Here's how the part is built. I have some questions about the finished solid (model axes, mm). Round coordinates to 2 decimals unless told otherwise and drop trailing zeros. Order: outer loops, then holes, each group sorted by start corner. A loop starts at its lowest first (then second) coordinate and runs counter-clockwise, first axis right, second up.
```python
from build123d import *

# Parameters (mm, degrees)
F1_DEPTH = 6.7056


# Not quite as in the source:
# - the program builds the solid bodies; features that only make, move or delete a surface that nothing else refers to are left out


with BuildPart() as f1:
    # F0 (on Front) → F1 (new body)
    with BuildSketch(Plane.XZ):
        with BuildLine():
            ThreePointArc((-32.0095643401, 38.8673432171), (-41.2789452821, 48.1367241591), (-50.5483262241, 38.8673432171))
            Line((-50.5483262241, 38.8673432171), (-50.5483262241, -38.9954559505))
            ThreePointArc((-50.5483262241, -38.9954559505), (-41.2789452821, -48.2648368925), (-32.0095643401, -38.9954559505))
            Line((-32.0095643401, -38.9954559505), (30.3480885923, -31.9170206785))
            ThreePointArc((30.3480885923, -31.9170206785), (49.5331583117, -22.4657405577), (58.3247691393, -2.9695569538))
            Line((58.3247691393, -2.9695569538), (58.3247691393, 3.3366130665))
            ThreePointArc((58.3247691393, 3.3366130665), (49.99023947, 23.5446765042), (30.3480885923, 33.1371799111))
            Line((30.3480885923, 33.1371799111), (-32.0095643401, 38.8673432171))
        make_face()
    extrude(amount=F1_DEPTH)


solid = f1.part
```
1) If we section it at B-B (x = 14): Write out the boundary of the cut face in (y, z).
2) I need wall thicknesses on line 1 (Z direction, x = -27, y = -1.75); line 2 (Z direction, x = -9, y = -6.25); line 3 (X direction, y = -0.25, z = 20). Which ranges of each line are inside material? Lowest first, please.
3) I'm going to push flat-ended pins straight in: pin 1 (1.5 mm diameter, centred on y = -5.5, z = 14.5, fed in from +X); pin 2 (4 mm diameter, centred on x = 18, y = -5.5, fed in from -Z). Where does each tip first touch, or does it pass through?
4) If we section it at A-A (y = -2.75): Write out the boundary of the cut face in (x, z).
5) We'd pull the mould along Y, two halves only. Please class faces 1 (the flat face through (-9, -6.706, 1)), 2 (the flat face through (-50.548, -3, 0)), 3 (the flat face through (-9, 0, 1)): +Y half, -Y half, draft (parallel to the pull), parting line (faces both ways), or undercut.
6) If we section it at C-C (z = -11): Write out the boundary of the cut face in (x, y), plus the area to 3 significant figures.
Solutions:
1. outline: (-6.71, -33.77) - (0, -33.77) - (0, 34.64) - (-6.71, 34.64) - close
2. line 1: z = -38.43 to 38.41
2. line 2: z = -36.38 to 36.75
2. line 3: x = -50.55 to 52.86
3. pin 1: stops at x = 56.19
3. pin 2: stops at z = -33.55
4. outline: (-50.55, -39) arc R9.27 ccw to (-32.01, -39) - (30.35, -31.92) arc R31.64 ccw to (58.32, -2.97) - (58.32, 3.34) arc R30.81 ccw to (30.35, 33.14) - (-32.01, 38.87) arc R9.27 ccw to (-50.55, 38.87) - close
5. face 1: -Y half
5. face 2: draft
5. face 3: +Y half
6. outline: (-50.55, -6.71) - (56.62, -6.71) - (56.62, 0) - (-50.55, 0) - close
6. area: 719 mm2
